Read the model definition and answer for the solid it produces. Units are mm, in the model's axes. Face numbers are marked on the shaded views. A direction names the side the tool comes from. Round coordinates to 2 decimals unless told otherwise and drop trailing zeros. Loops run counter-clockwise (first coordinate to the right, second up) from the corner with the lowest first, then second, coordinate; pieces in that order, holes last. Notation, with made-up numbers: M 54,-16.75 L 105,-16.75 A24 cw 105,7.25 Z; hole C 84.25,-21 d1. An arc over 180 degrees is marked long. Write each question's results on one line, items separated by ' | '.
from build123d import *

# Parameters (mm, degrees)
SKETCH1_R           = 3.6576
BOSS_EXTRUDE1_DEPTH = 4.1275
BOSS_EXTRUDE2_START = -35.56
SKETCH2_R           = 3.6576
BOSS_EXTRUDE2_DEPTH = 12.7
SKETCH3_R           = 6.1976
CUT_EXTRUDE1_DEPTH  = 72.691050043


with BuildPart() as part:
    # Sketch1 → Boss-Extrude1 (new body)
    with BuildSketch(Plane.XY):
        with BuildLine():
            Line((0, 0), (12.7, 0))
            ThreePointArc((12.7, 0), (17.190128061, 1.859871939), (19.05, 6.35))
            Line((19.05, 6.35), (19.05, 62.23))
            ThreePointArc((19.05, 62.23), (17.190128061, 66.720128061), (12.7, 68.58))
            Line((12.7, 68.58), (0, 68.58))
            Line((0, 68.58), (0, 0))
        make_face()
        with Locations((7.493, 60.96)):
            Circle(SKETCH1_R, mode=Mode.SUBTRACT)
        with Locations((7.493, 7.62)):
            Circle(SKETCH1_R, mode=Mode.SUBTRACT)
    extrude(amount=BOSS_EXTRUDE1_DEPTH)

    # Sketch2 → Boss-Extrude2 (add)
    with BuildSketch(Plane(origin=(0, 68.58, 0), x_dir=(1, 0, 0), z_dir=(0, 1, 0)).offset(BOSS_EXTRUDE2_START)):
        with BuildLine():
            Line((0, 0), (-6.35, 0))
            ThreePointArc((-6.35, 0), (-10.840128061, -10.840128061), (0, -6.35))
            Line((0, -6.35), (0, -4.1275))
            Line((0, -4.1275), (0, 0))
        make_face()
        with Locations(Location((-6.35, -6.35, 0), (0, 0, 270))):
            Circle(SKETCH2_R, mode=Mode.SUBTRACT)
    extrude(amount=-BOSS_EXTRUDE2_DEPTH)

    # Sketch3 → Cut-Extrude1 (cut, through all)
    with BuildSketch(Plane.XY.offset(4.1275)):
        with Locations((7.493, 46.99)):
            Circle(SKETCH3_R)
        with Locations((7.493, 21.59)):
            Circle(SKETCH3_R)
    extrude(amount=-CUT_EXTRUDE1_DEPTH, mode=Mode.SUBTRACT)


solid = part.part
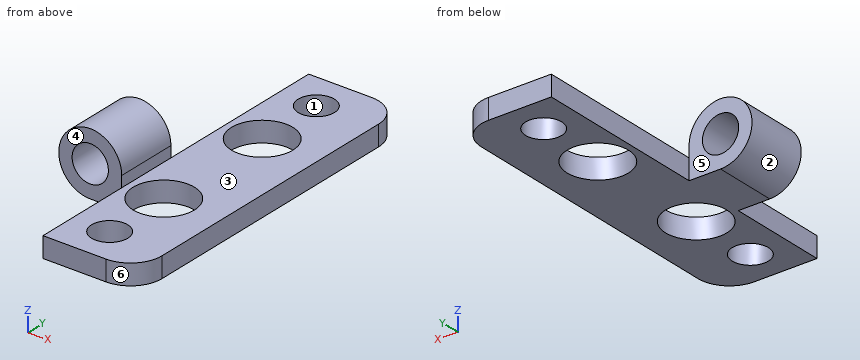
Item 1: The mould has two halves that part along X. Classify the marked faces 1, 2 and 3: pulls with the +X half, pulls with the -X half, needs draft (parallel to the pull), parting line crosses it, or undercut.
Outcome:
face 1: undercut | face 2: parting line crosses it | face 3: needs draft
Item 2: The part is cut by section A-A (y = 46.99). Determine the outline of the cut face in (x, z), plus the area to 3 significant figures.
Outcome:
outline: M 0,0 L 1.3,0 L 1.3,4.13 L 0,4.13 Z; M 13.69,0 L 19.05,0 L 19.05,4.13 L 13.69,4.13 Z | area: 27.5 mm2
Item 3: For the marked faces 4, 5 and 6, determine the directions among +Z, -Z, +X, -X, +Y, -Y from which every point of the face is accessible in a straight line to the end or side of a thin tool.
Outcome:
face 4: +Z, -Z, -X, -Y | face 5: +Z, -Z, -X, +Y | face 6: +Z, -Z, +X, -Y
Item 4: Straight lines are drawn through the part: line 1 (X direction, y = 29.75, z = 6.35); line 2 (X direction, y = 12, z = 2.25); line 3 (Y direction, x = -8, z = 10). For each, find the intervals that lie inside material, in ascending order.
Outcome:
line 1: x = -12.7 to -10.01, -2.69 to 0 | line 2: x = 0 to 19.05 | line 3: y = 20.32 to 33.02
Item 5: Flat-ended cylindrical pins translate along their axes: pin 1 (6.5 mm diameter, centred on x = -6, z = 8.5, fed in from +Y); pin 2 (1.2 mm diameter, centred on y = 9.5, z = 2, fed in from -X); pin 3 (11 mm diameter, centred on x = 7.493, y = 21.59, fed in from +Z); pin 4 (15 mm diameter, centred on x = 10, y = 30, fed in from +Z). Find the tip coordinate at first contact, or state that the pin passes through.
Outcome:
pin 1: stops at y = 33.02 | pin 2: stops at x = 0 | pin 3: passes through | pin 4: stops at z = 4.13
Item 6: The part is cut by section D-D (y = 54.5). Determine the outline of the cut face in (x, z), plus the area to 3 significant figures.
Outcome:
outline: M 0,0 L 19.05,0 L 19.05,4.13 L 0,4.13 Z | area: 78.6 mm2
Item 7: The part is cut by section C-C (x = 2). Determine the outline of the cut face in (y, z).
Outcome:
outline: M 0,0 L 18.72,0 L 18.72,4.13 L 0,4.13 Z; M 24.46,0 L 44.12,0 L 44.12,4.13 L 24.46,4.13 Z; M 49.86,0 L 68.58,0 L 68.58,4.13 L 49.86,4.13 Z
Item 8: The part is cut by section B-B (z = 9). Determine the outline of the cut face in (x, y), plus the area to 3 significant figures.
Outcome:
outline: M -12.12,20.32 L -8.87,20.32 L -8.87,33.02 L -12.12,33.02 Z; M -3.83,20.32 L -0.58,20.32 L -0.58,33.02 L -3.83,33.02 Z | area: 82.5 mm2
